Read the model definition and answer for the solid it produces. Units are mm, in the model's axes. A direction names the side the tool comes from. Coordinates: 2 decimals unless noted, no trailing zeros. Write each loop counter-clockwise with the first axis right and the second up, starting at its lowest first coordinate (ties: lowest second). Pieces come first, ordered by that corner, then holes.
Item 1: Each of these flat-tipped pins is pushed along its axis until it touches: P1, Ø1.6, axis at x = -16.37, y = -56.075, coming from the +Z side; P2, Ø10.5, axis at x = 19, y = -19, coming from the -Z side; P3, Ø5, axis at x = -19, y = 19, coming from the +Z side; P4, Ø16, axis at x = 8.5, z = 22, coming from the -Y side. Where does it stop, or does it pass through?
Item 2: A tool of negligible diameter and unlimited length cuts with its end or side. For faces 4 (the face through (-14.12, -49, -11)), 5 (the face through (21.4, -46.4, 1)), 6 (the face through (21, -50, 2)), from which of +Z, -Z, +X, -X, +Y, -Y can it reach the whole face along a straight path? Write none if from no direction.
Item 3: Determine the mould class of faces 1 (the face through (25, -49, 2)), 2 (the face through (-17, 19, 4)), 3 (the face through (-13.52, -48.99, -20.43)) for opening direction X: released by +X, released by -X, zero draft, split by the parting line, or undercut.
Item 4: Straight lines are drawn through the part: probe 1 along X at (y, z) = (29, 23); probe 2 along X at (y, z) = (-45, 0.35); probe 3 along Y at (x, z) = (-19, 2.15). For each, find the intervals that lie inside material, in ascending order.
Item 5: Section C-C (y = 11) is taken. Give the vertices of the cut face in (x, z), then the cut area to 3 significant figures.
Item 6: Section B-B (z = -7.5) is taken. Give the vertices of the cut face in (x, y).
Item 7: Section A-A (x = -4.5) is taken. Give the vertices of the cut face in (y, z).
from build123d import *

# Parameters (mm, degrees)
SKETCH_1_R               = 1.6
SKETCH_1_R_2             = 1.375
EXTRUDE_1_DEPTH          = 5
SKETCH_2_W               = 54
SKETCH_2_H               = 15
EXTRUDE_2_DEPTH          = 25
SKETCH_3_R               = 3
CUT_EXTRUDE_1_DEPTH      = 10
FILLET_1_R               = 7
FILLET_2_R               = 5
FILLET_3_R               = 5
CHAMFER_1_SIZE           = 0.5
CUT_EXTRUDE_2_DEPTH      = 73.226189886
CUT_EXTRUDE_2_DEPTH_BACK = 1
SKETCH_4_R               = 4
FILLET_4_R               = 5
SKETCH_5_W               = 23
SKETCH_5_H               = 4
EXTRUDE_3_DEPTH          = 21
FILLET_5_R               = 2
FILLET_6_R               = 3
CUT_EXTRUDE_3_DEPTH      = 1
CUT_EXTRUDE_3_DEPTH_BACK = 75.10548229
SKETCH_6_R               = 3.25


with BuildPart() as part:
    # 草图1 → 凸台-拉伸1 (new body)
    with BuildSketch(Plane.XY):
        Polygon((-27, -50), (-23.12, -50), (-19.12, -62.15), (-14.12, -62.15), (-14.12, -50), (8.88, -50), (8.88, -62.15), (13.88, -62.15), (17.88, -50), (27, -50), (27, 39), (-27, 39), align=None)
        with Locations((-19, 19)):
            Circle(SKETCH_1_R, mode=Mode.SUBTRACT)
        with Locations((19, 19)):
            Circle(SKETCH_1_R, mode=Mode.SUBTRACT)
        with Locations((19, -19)):
            Circle(SKETCH_1_R, mode=Mode.SUBTRACT)
        with Locations((-19, -19)):
            Circle(SKETCH_1_R, mode=Mode.SUBTRACT)
        with Locations((-20, -45)):
            Circle(SKETCH_1_R, mode=Mode.SUBTRACT)
        with Locations(Location((20, -45, 0), (0, 0, 180))):
            Circle(SKETCH_1_R, mode=Mode.SUBTRACT)
        with Locations((-16.37, -56.075)):
            Circle(SKETCH_1_R_2, mode=Mode.SUBTRACT)
        with Locations(Location((11.13, -56.075, 0), (0, 0, 180))):
            Circle(SKETCH_1_R_2, mode=Mode.SUBTRACT)
    extrude(amount=EXTRUDE_1_DEPTH)

    # 草图2 → 凸台-拉伸2 (add)
    with BuildSketch(Plane.XY.offset(5)):
        with Locations((0, 31.5)):
            Rectangle(SKETCH_2_W, SKETCH_2_H)
    extrude(amount=EXTRUDE_2_DEPTH)

    # 草图3 → 切除-拉伸1 (cut)
    with BuildSketch(Plane.XZ.offset(-24)):
        with Locations(Location((-20, 23, 0), (0, 0, 270))):
            Circle(SKETCH_3_R)
        with Locations(Location((20, 23, 0), (0, 0, 90))):
            Circle(SKETCH_3_R)
    extrude(amount=-CUT_EXTRUDE_1_DEPTH, mode=Mode.SUBTRACT)

    # 圆角1
    fillet_1_edges = [part.edges().sort_by_distance(p)[0] for p in [
        (-27, 31.5, 30),
        (27, 31.5, 30),
    ]]
    fillet(fillet_1_edges, radius=FILLET_1_R)

    # 圆角2
    fillet_2_edges = [part.edges().sort_by_distance(p)[0] for p in [
        (0, 39, 30),
        (-27, 39, 11.5),
        (27, 39, 11.5),
        (-24.949747468, 39, 27.949747468),
        (24.949747468, 39, 27.949747468),
    ]]
    fillet(fillet_2_edges, radius=FILLET_2_R)

    # 圆角3
    # the kernel refuses this fillet: 5 mm, written as the material it adds along each edge
    with BuildSketch(Plane(origin=(27, 24, 5), x_dir=(0, 0, 1), z_dir=(-1, 0, 0))) as fillet_3_piece_1_section:
        with BuildLine():
            CenterArc((FILLET_3_R, -FILLET_3_R), FILLET_3_R, 90, 90)
            Line((0, -FILLET_3_R), (0, 0))
            Line((0, 0), (FILLET_3_R, 0))
        make_face()
    fillet_3_piece_1 = extrude(amount=54, mode=Mode.PRIVATE)
    fillet_3_piece_1 = fillet_3_piece_1 - Plane(origin=(-19, 19, 6.136368117), x_dir=(1, 0, 0), z_dir=(0, 0, -1)) * Cylinder(1.6, 128, mode=Mode.PRIVATE)
    fillet_3_piece_1 = fillet_3_piece_1 - Plane(origin=(19, 19, 6.136368117), x_dir=(1, 0, 0), z_dir=(0, 0, -1)) * Cylinder(1.6, 128, mode=Mode.PRIVATE)
    add(fillet_3_piece_1)

    # 倒角1
    chamfer_1_edges = [part.edges().sort_by_distance(p)[0] for p in [
        (-20, 24, 26),
        (20, 24, 20),
    ]]
    chamfer(chamfer_1_edges, length=CHAMFER_1_SIZE)

    # 草图4 → 切除-拉伸2 (cut, two sides: drawn at the far end of the back side and taken through both)
    with BuildSketch(Plane.XY.offset(5).offset(-CUT_EXTRUDE_2_DEPTH_BACK)):
        with Locations((-19, 19)):
            Circle(SKETCH_4_R)
        with Locations((19, 19)):
            Circle(SKETCH_4_R)
        with Locations(Location((-19, -19, 0), (0, 0, 180))):
            Circle(SKETCH_4_R)
        with Locations(Location((19, -19, 0), (0, 0, 180))):
            Circle(SKETCH_4_R)
    extrude(amount=CUT_EXTRUDE_2_DEPTH + CUT_EXTRUDE_2_DEPTH_BACK, mode=Mode.SUBTRACT)

    # 圆角4
    # the kernel refuses this fillet: 5 mm, written as the material it takes off along each edge
    with BuildSketch(Plane(origin=(27, -50, -12.5), x_dir=(0, 1, 0), z_dir=(0, 0, 1))) as fillet_4_piece_1:
        with BuildLine():
            CenterArc((FILLET_4_R, FILLET_4_R), FILLET_4_R, 180, 90)
            Line((0, FILLET_4_R), (-FILLET_4_R * 0.02, FILLET_4_R))
            Line((-FILLET_4_R * 0.02, FILLET_4_R), (-FILLET_4_R * 0.02, -FILLET_4_R * 0.02))
            Line((-FILLET_4_R * 0.02, -FILLET_4_R * 0.02), (FILLET_4_R, -FILLET_4_R * 0.02))
            Line((FILLET_4_R, -FILLET_4_R * 0.02), (FILLET_4_R, 0))
        make_face()
    extrude(amount=30, mode=Mode.SUBTRACT)
    with BuildSketch(Plane(origin=(-27, -50, -12.182364303), x_dir=(0, 1, 0), z_dir=(0, 0, 1))) as fillet_4_piece_2:
        with BuildLine():
            CenterArc((4.872945721, -5), FILLET_4_R, 90, 77.055918457)
            Line((0, -3.88), (-0.097458914, -3.8576))
            ThreePointArc((-0.097458914, -3.8576), (-0.1, -1.94), (-0.1, 0))
            Line((-0.1, 0), (0, 0.1))
            Line((0, 0.1), (4.872945721, 0.1))
            Line((4.872945721, 0.1), (4.872945721, 0))
        make_face()
    extrude(amount=29.364728605, mode=Mode.SUBTRACT)

    # 草图5 → 凸台-拉伸3 (add)
    with BuildSketch(Plane(origin=(0, 0, 0), x_dir=(-1, 0, 0), z_dir=(0, 0, -1))):
        with Locations((2.62, -48)):
            Rectangle(SKETCH_5_W, SKETCH_5_H)
    extrude(amount=EXTRUDE_3_DEPTH)

    # 圆角5
    fillet_5_edges = [part.edges().sort_by_distance(p)[0] for p in [
        (8.88, -46, -10.5),
        (-14.12, -46, -10.5),
        (8.88, -48, -21),
        (-14.12, -48, -21),
        (-2.62, -46, -21),
        (17.88, -50, 2.5),
        (13.88, -62.15, 2.5),
        (-19.12, -62.15, 2.5),
        (-23.12, -50, 2.5),
    ]]
    fillet(fillet_5_edges, radius=FILLET_5_R)

    # 圆角6
    fillet_6_edges = [part.edges().sort_by_distance(p)[0] for p in [
        (-14.12, -49, 0),
        (8.88, -49, 0),
        (-2.62, -46, 0),
        (8.294213562, -46.585786438, 0),
        (-13.534213562, -46.585786438, 0),
    ]]
    fillet(fillet_6_edges, radius=FILLET_6_R)

    # 草图6 → 切除-拉伸3 (cut, two sides: drawn at the far end of the back side and taken through both)
    with BuildSketch(Plane.XY.offset(-CUT_EXTRUDE_3_DEPTH_BACK)):
        with Locations((-20, -45)):
            Circle(SKETCH_6_R)
        with Locations((20, -45)):
            Circle(SKETCH_6_R)
    extrude(amount=CUT_EXTRUDE_3_DEPTH + CUT_EXTRUDE_3_DEPTH_BACK, mode=Mode.SUBTRACT)


solid = part.part
Established:
1. P1: passes through
1. P2: stops at z = 0
1. P3: stops at z = 4
1. P4: stops at y = 24
2. face 4: -Z, -X, +Y, -Y
2. face 5: -Z
2. face 6: +Z, -Z, +X, -Y
3. face 1: released by +X
3. face 2: undercut
3. face 3: released by -X
4. probe 1: x = -27 to -23, -17 to 17, 23 to 27
4. probe 2: x = -27 to -23.25, -16.75 to 16.75, 23.25 to 27
4. probe 3: y = -61.65 to -46.25, -43.75 to -20.6, -17.4 to 17.4, 20.6 to 39
5. outline: (-27, 0) - (27, 0) - (27, 5) - (-27, 5) - close
5. area: 270 mm2
6. outline: (-14.12, -50) - (8.88, -50) - (8.88, -48) arc R2 ccw to (6.88, -46) - (-12.12, -46) arc R2 ccw to (-14.12, -48) - close
7. outline: (-50, -21) - (-48, -21) arc R2 ccw to (-46, -19) - (-46, -3) arc R3 cw to (-43, 0) - (39, 0) - (39, 25) arc R5 ccw to (34, 30) - (24, 30) - (24, 10) arc R5 cw to (19, 5) - (-50, 5) - close
